Answer from the drawing. Dimensions are ordinates in mm from the lowest x, y and z of the part. A direction names the side the tool comes from. Give positions to 0.01 mm unless a question says otherwise; leave off trailing zeros. Order: outer loops, then holes, each group sorted by start corner. A loop starts at its lowest first (then second) coordinate and runs counter-clockwise, first axis right, second up. Notation, with made-up numbers: (17.5, 68.5) - (43.5, 68.5) arc R10 ccw to (43.5, 85.5) - close; hole circle Ø11 at (51, 63.5). An arc over 180 degrees is marked (long way). Write each question's results on one line, items separated by ' | '.
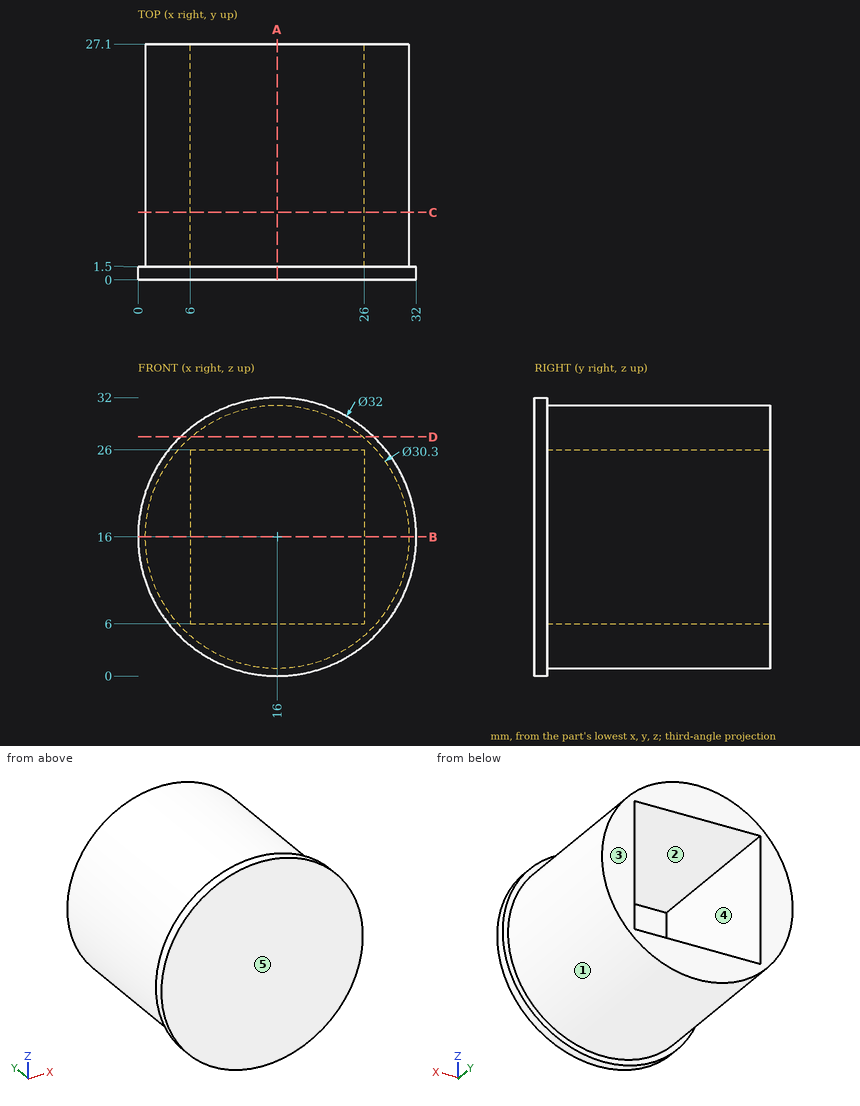
1. A cutting plane is placed at B-B, the plane z = 16. Write down the section's boundary in (x, y), then the cut area to 3 significant figures.
Answer list:
outline: (0, 0) - (32, 0) - (32, 1.5) - (31.15, 1.5) - (31.15, 27.1) - (26, 27.1) - (26, 1.5) - (6, 1.5) - (6, 27.1) - (0.85, 27.1) - (0.85, 1.5) - (0, 1.5) - close | area: 312 mm^2
2. Given P1, Ø1, axis at y = 4, z = 3, coming from the +X side; P2, Ø1.5, axis at y = 14, z = 25, coming from the +X side; P3, Ø16, axis at y = 18, z = 12, coming from the +X side; P4, Ø8, axis at x = 6.5, z = 16.5, coming from the -Y side, each flat-ended and moving along its own axis, determine where each tip first touches the part or whether it passes through.
Answer list:
P1: x = 24.56 | P2: x = 28.71 | P3: x = 31.15 | P4: y = 0
3. Straight lines are drawn through the part: line 1 (Y direction, x = 25.5, z = 9); line 2 (X direction, y = 1.75, z = 16); line 3 (X direction, y = 19, z = 10). For each, find the intervals that lie inside material, in ascending order. Write a range as [from, to].
Answer list:
line 1: [0, 1.5] | line 2: [0.85, 6], [26, 31.15] | line 3: [2.09, 6], [26, 29.91]
4. A tool of negligible diameter and unlimited length cuts with its end or side. For the marked faces 4 and 5, from which of +Z, -Z, +X, -X, +Y, -Y can it reach the whole face along a straight path? Write none if from no direction.
Answer list:
face 4: +Y | face 5: +Z, -Z, +X, -X, -Y
5. A cutting plane is placed at D-D, the plane z = 27.5. Write down the section's boundary in (x, y).
Answer list:
outline: (4.88, 0) - (27.12, 0) - (27.12, 1.5) - (25.86, 1.5) - (25.86, 27.1) - (6.14, 27.1) - (6.14, 1.5) - (4.88, 1.5) - close
6. Determine the mould class of the marked faces 1, 2 and 3 for opening direction Z: +Z half, -Z half, draft (parallel to the pull), parting line (faces both ways), or undercut.
Answer list:
face 1: parting line | face 2: undercut | face 3: draft
7. A cutting plane is placed at C-C, the plane y = 7.75. Write down the section's boundary in (x, z).
Answer list:
outline: circle Ø30.3 at (16, 16); hole (6, 6) - (26, 6) - (26, 26) - (6, 26) - close
8. A cutting plane is placed at A-A, the plane x = 16. Write down the section's boundary in (y, z).
Answer list:
outline: (0, 0) - (1.5, 0) - (1.5, 0.85) - (27.1, 0.85) - (27.1, 6) - (1.5, 6) - (1.5, 26) - (27.1, 26) - (27.1, 31.15) - (1.5, 31.15) - (1.5, 32) - (0, 32) - close
